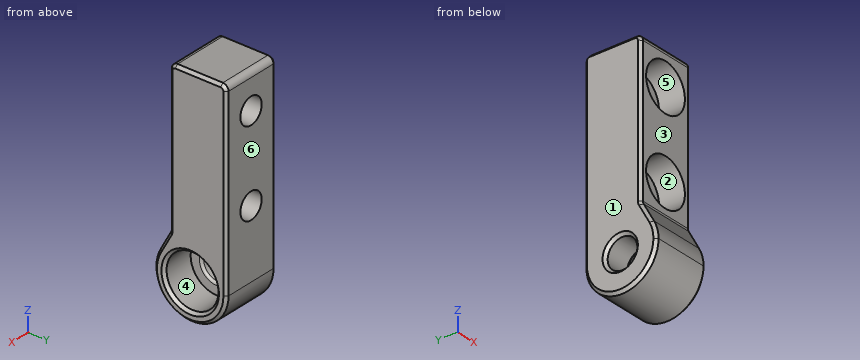
```python
from build123d import *

# Parameters (mm, degrees)
SKETCH5_R                               = 3.15
BOSS_EXTRUDE5_DEPTH                     = 12.8
CBORE_FOR_M5_HEX_HEAD_BOLT1_D           = 5.5
CBORE_FOR_M5_HEX_HEAD_BOLT1_CBORE_D     = 10
CBORE_FOR_M5_HEX_HEAD_BOLT1_CBORE_DEPTH = 5.5
SKETCH8_R                               = 5.5
CUT_EXTRUDE_LEFT_DEPTH                  = 6.8
FILLET5_R                               = 1.2
CHAMFER2_SIZE                           = 0.6
FILLET7_R                               = 0.5


with BuildPart() as part:
    # Sketch5 → Boss-Extrude5 (new body)
    with BuildSketch(Plane(origin=(0, 0, 0), x_dir=(0, -1, 0), z_dir=(1, 0, 0))):
        with BuildLine():
            Line((-7.65, 0), (-7.65, -40))
            Line((-7.65, -40), (4.35, -40))
            Line((4.35, -40), (4.35, -8))
            Line((4.35, -8), (6.715651055, -3.663677239))
            ThreePointArc((6.715651055, -3.663677239), (7.412733321, -1.890472088), (7.65, 0))
            ThreePointArc((7.65, 0), (0, 7.65), (-7.65, 0))
        make_face()
        Circle(SKETCH5_R, mode=Mode.SUBTRACT)
    extrude(amount=BOSS_EXTRUDE5_DEPTH)

    # CBORE for M5 Hex Head Bolt1 (through all)
    with Locations(Plane(origin=(0, -4.35, 0), x_dir=(-1, 0, 0), z_dir=(0, -1, 0))):
        with Locations((-6.4, -14.5), (-6.4, -32.5)):
            CounterBoreHole(CBORE_FOR_M5_HEX_HEAD_BOLT1_D / 2, CBORE_FOR_M5_HEX_HEAD_BOLT1_CBORE_D / 2, CBORE_FOR_M5_HEX_HEAD_BOLT1_CBORE_DEPTH)

    # Sketch8 → Cut-Extrude-LEFT (cut)
    with BuildSketch(Plane(origin=(12.8, 0, 0), x_dir=(0, 0, -1), z_dir=(1, 0, 0))):
        Circle(SKETCH8_R)
    extrude(amount=-CUT_EXTRUDE_LEFT_DEPTH, mode=Mode.SUBTRACT)

    # Fillet5
    fillet5_edges = [part.edges().sort_by_distance(p)[0] for p in [
        (6.4, -4.35, 40),
        (6.4, 7.65, 40),
        (6.4, -4.35, 8),
    ]]
    fillet(fillet5_edges, radius=FILLET5_R)

    # Chamfer2
    chamfer2_edges = [part.edges().sort_by_distance(p)[0] for p in [
        (12.8, -1.890472088, -7.412733321),
        (0, 3.15, 0),
        (12.8, 7.65, 19.4),
        (12.8, 0, 5.5),
        (0, -5.606107798, 5.697509604),
        (12.8, -5.606107798, 5.697509604),
        (0, -4.35, 23.553018219),
        (12.8, -4.35, 23.553018219),
        (0, 1.65, 40),
        (12.8, 1.65, 40),
        (0, -3.998528137, 39.648528137),
        (0, 7.298528137, 39.648528137),
        (12.8, -3.998528137, 39.648528137),
        (12.8, 7.298528137, 39.648528137),
        (0, -4.387218303, 8.009491797),
        (12.8, -4.387218303, 8.009491797),
        (0, 7.65, 19.4),
        (0, -1.890472088, -7.412733321),
    ]]
    chamfer(chamfer2_edges, length=CHAMFER2_SIZE)

    # Fillet7
    fillet7_edges = [part.edges().sort_by_distance(p)[0] for p in [
        (6, 3.15, 0),
    ]]
    fillet(fillet7_edges, radius=FILLET7_R)


solid = part.part
```
The model under review builds one solid part; all positions refer to its coordinate system, in mm. Face numbers are marked on the shaded views. A direction names the side the tool comes from. Give positions to 0.01 mm unless a question says otherwise; leave off trailing zeros. Loops run counter-clockwise (first coordinate to the right, second up) from the corner with the lowest first, then second, coordinate; pieces in that order, holes last. Notation, with made-up numbers: (-17.75, 75.5) - (-3.75, 75.5) arc R13 cw to (-3.75, 84.5) - close; hole circle Ø10 at (-24, 8.5). An arc over 180 degrees is marked (long way). Answer as a JSON object with one key per item and string values.
Q1. For the marked faces 1, 2 and 3, list the 3-axis set-ups (+Z, -Z, +X, -X, +Y, -Y) from which the entire face can be reached by the end or side of a thin tool; tool diameter is ignored.
Worked out:
{"face 1": "+Z, -Z, -X, +Y, -Y", "face 2": "-Y", "face 3": "+Z, +X, -X, -Y"}
Q2. Add section A-A on y = 0. State the section outline as (x, z) points.
Worked out:
{"outline": "(0, -7.05) - (0.6, -7.65) - (12.2, -7.65) - (12.8, -7.05) - (12.8, -6.1) - (12.2, -5.5) - (6, -5.5) - (6, -3.65) arc R0.5 ccw to (5.5, -3.15) - (0.6, -3.15) - (0, -3.75) - close; (0, 3.75) - (0.6, 3.15) - (5.5, 3.15) arc R0.5 ccw to (6, 3.65) - (6, 5.5) - (12.2, 5.5) - (12.8, 6.1) - (12.8, 39.4) - (12.2, 40) - (0.6, 40) - (0, 39.4) - close; hole circle Ø10 at (6.4, 14.5); hole circle Ø10 at (6.4, 32.5)"}
Q3. Insertion check: pin 1 (3 mm diameter, centred on x = 6.5, z = 34, fed in from -Y); pin 2 (5 mm diameter, centred on x = 6.4, z = 32.5, fed in from -Y); pin 3 (3 mm diameter, centred on x = 7, z = 3, fed in from -Y); pin 4 (2 mm diameter, centred on y = -5.5, z = -1.5, fed in from +X). Each pin has a flat end and moves straight along its axis. Give the tip position at first contact, or say it passes through.
Worked out:
{"pin 1": "stops at y = 1.15", "pin 2": "passes through", "pin 3": "stops at y = -7.5", "pin 4": "stops at x = 12.8"}
Q4. Mouldability with a two-part tool opening along Y and no side actions: class the marked faces 4, 5 and 6 as +Y half, -Y half, draft (parallel to the pull), parting line (faces both ways), or undercut.
Worked out:
{"face 4": "undercut", "face 5": "draft", "face 6": "+Y half"}
Q5. Add section C-C on x = 9.75. State the section outline as (y, z) points, plus the area to 3 significant figures.
Worked out:
{"outline": "(-6.72, 3.66) arc R7.65 ccw (long way) to (7.65, 0) - (7.65, 38.8) arc R1.2 ccw to (6.45, 40) - (-3.15, 40) arc R1.2 ccw to (-4.35, 38.8) - (-4.35, 36.21) - (1.15, 36.21) - (1.15, 28.79) - (-4.35, 28.79) - (-4.35, 18.21) - (1.15, 18.21) - (1.15, 10.79) - (-4.35, 10.79) - (-4.35, 8.31) arc R1.2 cw to (-4.5, 7.73) - close; hole circle Ø11 at (0, 0)", "area": "411 mm^2"}
Q6. Add section D-D on z = 22. State the section outline as (x, y) points, plus the area to 3 significant figures.
Worked out:
{"outline": "(0, -3.75) - (0.6, -4.35) - (12.2, -4.35) - (12.8, -3.75) - (12.8, 7.05) - (12.2, 7.65) - (0.6, 7.65) - (0, 7.05) - close", "area": "153 mm^2"}
Q7. Add section B-B on z = 32.5. State the section outline as (x, y) points.
Worked out:
{"outline": "(0, -3.75) - (0.6, -4.35) - (1.4, -4.35) - (1.4, 1.15) - (3.65, 1.15) - (3.65, 7.65) - (0.6, 7.65) - (0, 7.05) - close; (9.15, 1.15) - (11.4, 1.15) - (11.4, -4.35) - (12.2, -4.35) - (12.8, -3.75) - (12.8, 7.05) - (12.2, 7.65) - (9.15, 7.65) - close"}
Q8. To check wall thickness, follow line 1 along Z through (x, y) = (6.4, -2.45); line 2 along Z through (x, y) = (3.45, 0); line 3 along Y through (x, z) = (10.75, 0). State the ranges of each line that lie inside material, in increasing order.
Worked out:
{"line 1": "z = -7.25 to -4.92, 4.92 to 9.5, 19.5 to 27.5, 37.5 to 40", "line 2": "z = -7.65 to -3.15, 3.15 to 10.46, 18.54 to 28.46, 36.54 to 40", "line 3": "y = -7.65 to -5.5, 5.5 to 7.65"}
